Part model, mm, in its own coordinate system. Coordinates: 2 decimals unless noted, no trailing zeros. Loops run counter-clockwise (first coordinate to the right, second up) from the corner with the lowest first, then second, coordinate; pieces in that order, holes last. Notation, with made-up numbers: (71, 59.5) -> (104, 59.5) arc R11 cw to (104, 64.5) -> close; hole circle Ø4 at (40, 1). An arc over 180 degrees is marked (long way). One line per item, written item: value. Start each with the question number.
from build123d import *

# Parameters (mm, degrees)
UTILITY_CIRCULAR_CROSS_SECTION_R   = 1.75
UTILITY_CIRCULAR_CROSS_SECTION_R_2 = 0.6


with BuildPart() as part:
    # Native hollow utility sweep: sweep along a path in Illustrative smooth utility route
    with BuildLine(Plane(origin=(0, 0, 0), x_dir=(0, 0, -1), z_dir=(1, 0, 0))) as native_hollow_utility_sweep_path:
        Line((-16.25, 0), (-16.25, -6))
        ThreePointArc((-16.25, -6), (-14.702430847, -12.680486977), (-10.375, -18))
        ThreePointArc((-10.375, -18), (-6.047569153, -23.319513023), (-4.5, -30))
        Line((-4.5, -30), (-4.5, -266))
    # Utility circular cross section → Native hollow utility sweep (sweep)
    with BuildSketch(Plane(origin=(0, 0, 0), x_dir=(1, 0, 0), z_dir=(0, 1, 0))):
        with Locations((0, -16.25)):
            Circle(UTILITY_CIRCULAR_CROSS_SECTION_R)
        with Locations((0, -16.25)):
            Circle(UTILITY_CIRCULAR_CROSS_SECTION_R_2, mode=Mode.SUBTRACT)
    sweep(path=native_hollow_utility_sweep_path.line)


solid = part.part
1) Slice it at A-A (x = 0). Give the cut face in (y, z).
2) Slice it at B-B (y = -62.5). Give the cut face in (x, z).
3) Probe line 1 (Z direction, x = 0, y = -147); line 2 (Z direction, x = 0, y = -3.55); line 3 (X direction, y = -246, z = 5). List the from-to ranges inside material, lowest first. Write a range as from..to.
4) Pin check, flat tips, straight feed: pin 1 Ø8 at (y, z) = (-153.5, 8) entering from -X; pin 2 Ø1.5 at (x, y) = (-1, -45) entering from +Z; pin 3 Ø1.4 at (x, z) = (0, 16.25) entering from -Y. Stop position of each tip, or through.
Check sheet entries:
1. outline: (-266, 2.75) -> (-30, 2.75) arc R16.94 ccw to (-16.62, 9.3) arc R13.44 cw to (-6, 14.5) -> (0, 14.5) -> (0, 15.65) -> (-6, 15.65) arc R14.59 ccw to (-17.53, 10.01) arc R15.79 cw to (-30, 3.9) -> (-266, 3.9) -> close; (-266, 5.1) -> (-30, 5.1) arc R14.59 ccw to (-18.47, 10.74) arc R15.79 cw to (-6, 16.85) -> (0, 16.85) -> (0, 18) -> (-6, 18) arc R16.94 ccw to (-19.38, 11.45) arc R13.44 cw to (-30, 6.25) -> (-266, 6.25) -> close
2. outline: circle Ø3.5 at (0, 4.5); hole circle Ø1.2 at (0, 4.5)
3. line 1: z = 2.75..3.9, 5.1..6.25
3. line 2: z = 14.5..15.65, 16.85..18
3. line 3: x = -1.68..-0.33, 0.33..1.68
4. pin 1: stops at x = -1.75
4. pin 2: stops at z = 6.23
4. pin 3: stops at y = -14.78
